Could you check a few things on this model? Use its own coordinates, in mm. Give positions to 0.01 mm unless a question says otherwise; leave off trailing zeros. Loops run counter-clockwise (first coordinate to the right, second up) from the corner with the lowest first, then second, coordinate; pieces in that order, holes last. Notation, with made-up numbers: (41.25, 69.25) - (80.25, 69.25) arc R10 cw to (80.25, 84.25) - close; hole circle Ø3 at (42, -16.5). An arc over 180 degrees is marked (long way). Write each question's results on one line, items separated by ' | '. Start each with the question number.
1) I want a section at B-B, the plane x = 8.5. Write out the boundary of the cut face in (y, z), and give its area (3 significant figures).
2) I want a section at C-C, the plane y = 5.5. Write out the boundary of the cut face in (x, z), and give its area (3 significant figures).
3) I want a section at D-D, the plane z = -14. Write out the boundary of the cut face in (x, y), and give its area (3 significant figures).
4) I'm going to push flat-ended pins straight in: pin 1 (5 mm diameter, centred on x = 6.5, z = -13.5, fed in from -Y); pin 2 (1.5 mm diameter, centred on x = 8.5, y = 3, fed in from -Z). Where does each tip first touch, or does it pass through?
5) I want a section at A-A, the plane y = 3. Write out the boundary of the cut face in (x, z), and give its area (3 significant figures).
6) If I drill on probe 1 along Y at (x, z) = (8.5, -20); probe 2 along Z at (x, y) = (3.25, 3.2); probe 3 along Z at (x, y) = (3.75, 2.9), over which ranges is the centre line in solid material (lowest first)? Write a range as [from, to].
from build123d import *

# Parameters (mm, degrees)
BOSS_EXTRUDE1_DEPTH = 6
SKETCH2_R           = 1.25
CUT_EXTRUDE1_DEPTH  = 31.245600159


with BuildPart() as part:
    # Sketch1 → Boss-Extrude1 (new body)
    with BuildSketch(Plane(origin=(0, 0, 0), x_dir=(1, 0, 0), z_dir=(0, 1, 0))):
        with BuildLine():
            Line((5.5, 27.323), (2.75, 27.323))
            Line((2.75, 27.323), (2.75, 22.092))
            ThreePointArc((2.75, 22.092), (3.88137085, 21.62337085), (4.35, 20.492))
            ThreePointArc((4.35, 20.492), (3.88137085, 19.36062915), (2.75, 18.892))
            Line((2.75, 18.892), (2.75, 13.6615))
            Line((2.75, 13.6615), (2.75, 8.431))
            ThreePointArc((2.75, 8.431), (3.88137085, 7.96237085), (4.35, 6.831))
            ThreePointArc((4.35, 6.831), (3.88137085, 5.69962915), (2.75, 5.231))
            Line((2.75, 5.231), (2.75, 0))
            Line((2.75, 0), (11.5, 0))
            Line((11.5, 0), (11.5, 27.323))
            Line((11.5, 27.323), (5.5, 27.323))
        make_face()
        with BuildLine():
            Line((2.75, 27.323), (0, 27.323))
            Line((0, 27.323), (0, 0))
            Line((0, 0), (2.75, 0))
            Line((2.75, 0), (2.75, 5.231))
            ThreePointArc((2.75, 5.231), (1.15, 6.831), (2.75, 8.431))
            Line((2.75, 8.431), (2.75, 13.6615))
            Line((2.75, 13.6615), (2.75, 18.892))
            ThreePointArc((2.75, 18.892), (1.15, 20.492), (2.75, 22.092))
            Line((2.75, 22.092), (2.75, 27.323))
        make_face()
    extrude(amount=BOSS_EXTRUDE1_DEPTH)

    # Sketch2 → Cut-Extrude1 (cut, through all)
    with BuildSketch(Plane.XY):
        with Locations((8.5, 3)):
            Circle(SKETCH2_R)
    extrude(amount=-CUT_EXTRUDE1_DEPTH, mode=Mode.SUBTRACT)


solid = part.part
Answers:
1) outline: (0, -27.32) - (1.75, -27.32) - (1.75, 0) - (0, 0) - close; (4.25, -27.32) - (6, -27.32) - (6, 0) - (4.25, 0) - close | area: 95.6 mm2
2) outline: (0, -27.32) - (11.5, -27.32) - (11.5, 0) - (0, 0) - close; hole circle Ø3.2 at (2.75, -20.49); hole circle Ø3.2 at (2.75, -6.83) | area: 298 mm2
3) outline: (0, 0) - (11.5, 0) - (11.5, 6) - (0, 6) - close; hole circle Ø2.5 at (8.5, 3) | area: 64.1 mm2
4) pin 1: stops at y = 0 | pin 2: passes through
5) outline: (0, -27.32) - (7.25, -27.32) - (7.25, 0) - (0, 0) - close; (9.75, -27.32) - (11.5, -27.32) - (11.5, 0) - (9.75, 0) - close; hole circle Ø3.2 at (2.75, -20.49); hole circle Ø3.2 at (2.75, -6.83) | area: 230 mm2
6) probe 1: y = [0, 1.75], [4.25, 6] | probe 2: z = [-27.32, -22.01], [-18.97, -8.35], [-5.31, 0] | probe 3: z = [-27.32, -21.74], [-19.24, -8.08], [-5.58, 0]
